Check sheet for the modelled part. Datum: model origin and axes. Units: mm. Round coordinates to 2 decimals unless told otherwise and drop trailing zeros. Write each loop counter-clockwise with the first axis right and the second up, starting at its lowest first coordinate (ties: lowest second). Pieces come first, ordered by that corner, then holes. Notation, with made-up numbers: (69.25, 30.25) -> (90.25, 30.25) arc R9 cw to (90.25, 46.25) -> close; hole circle Ø9 at (-7, 78.5). An arc over 180 degrees is marked (long way). Answer as a JSON object with one key per item and string values. Group by question number.
```python
from build123d import *

# Parameters (mm, degrees)
ESQUISSE1_R      = 8.25
ESQUISSE1_R_2    = 2
EXTRUSION1_DEPTH = 0.75
CONG_1_R         = 0.2


with BuildPart() as part:
    # Esquisse1 → Extrusion1 (new body)
    with BuildSketch(Plane.XY):
        Circle(ESQUISSE1_R)
        Circle(ESQUISSE1_R_2, mode=Mode.SUBTRACT)
    extrude(amount=EXTRUSION1_DEPTH)

    # Congé1
    cong_1_edges = [part.edges().sort_by_distance(p)[0] for p in [
        (-8.25, 0, 0),
        (-8.25, 0, 0.75),
        (-2, 0, 0),
        (-2, 0, 0.75),
    ]]
    fillet(cong_1_edges, radius=CONG_1_R)


solid = part.part
```
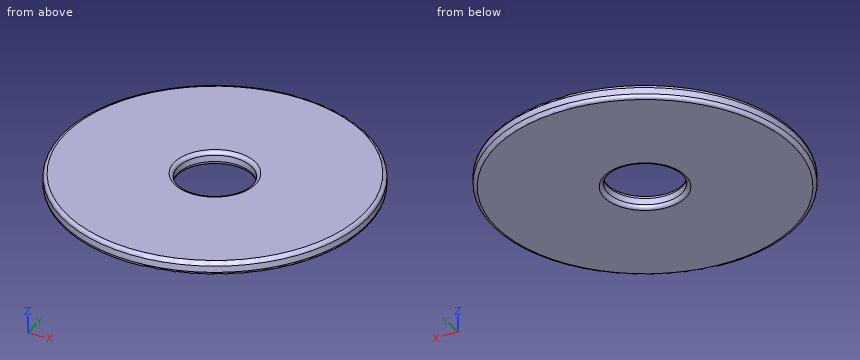
(1) Scan lines: line 1 along Y through (x, z) = (0, 0.4); line 2 along X through (y, z) = (-0.5, 0.6); line 3 along Y through (x, z) = (-1.5, 0.6). Record each from-to range of solid material in increasing order.
(2) Section check A-A on x = 0. Record the cut outline in (y, z).
Data:
{
 "1": {"line 1": "y = -8.25 to -2, 2 to 8.25", "line 2": "x = -8.23 to -1.94, 1.94 to 8.23", "line 3": "y = -8.11 to -1.33, 1.33 to 8.11"},
 "2": {"outline": "(-8.25, 0.2) arc R0.2 ccw to (-8.05, 0) -> (-2.2, 0) arc R0.2 ccw to (-2, 0.2) -> (-2, 0.55) arc R0.2 ccw to (-2.2, 0.75) -> (-8.05, 0.75) arc R0.2 ccw to (-8.25, 0.55) -> close; (2, 0.2) arc R0.2 ccw to (2.2, 0) -> (8.05, 0) arc R0.2 ccw to (8.25, 0.2) -> (8.25, 0.55) arc R0.2 ccw to (8.05, 0.75) -> (2.2, 0.75) arc R0.2 ccw to (2, 0.55) -> close"}
}
